For this review, take the finished solid that the model builds, in its own axes (mm). Face numbers are marked on the shaded views. Give positions to 0.01 mm unless a question says otherwise; leave off trailing zeros. Loops run counter-clockwise (first coordinate to the right, second up) from the corner with the lowest first, then second, coordinate; pieces in that order, holes last. Notation, with made-up numbers: (70.25, 44) - (85.25, 44) arc R22 ccw to (85.25, 61) - close; hole circle Ø6 at (13.25, 10.25). An arc over 180 degrees is marked (long way). Answer in a Markdown table with one row per item.
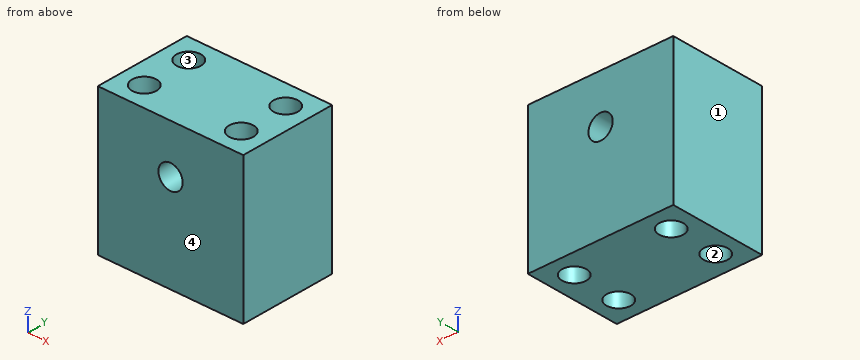
Autodesk Inventor part; units mm, degrees
ref_plane "YZ Plane" through (0, 0, 0) normal (1, 0, 0) x (0, 1, 0)
ref_plane "XZ Plane" through (0, 0, 0) normal (0, 1, 0) x (-1, 0, 0)
ref_plane "XY Plane" through (0, 0, 0) normal (0, 0, 1) x (1, 0, 0)
sketch "Sketch1" plane through (0, 0, 0) normal (0, 0, 1) x (1, 0, 0)
  line L0 (-19.05, -12.7) -> (19.05, -12.7)
  line L1 (19.05, -12.7) -> (19.05, 12.7)
  line L2 (19.05, 12.7) -> (-19.05, 12.7)
  line L3 (-19.05, 12.7) -> (-19.05, -12.7)
  line L4 (-19.05, -12.7) -> (19.05, 12.7) construction
  line L5 (19.05, -12.7) -> (-19.05, 12.7) construction
  point P0 (0, 0)
  dimension "d0" = 38.1
  dimension "d1" = 25.4
extrude "Extrusion1" add sketch "Sketch1" along normal blind 38.1
sketch "Sketch2" plane through (0, 0, 38.1) normal (0, 0, 1) x (1, 0, 0)
  line L0 (12.7, -6.35) -> (-12.7, -6.35)
  line L1 (-12.7, -6.35) -> (-12.7, 6.35)
  line L2 (-12.7, 6.35) -> (12.7, 6.35)
  line L3 (12.7, 6.35) -> (12.7, -6.35)
  line L4 (12.7, -6.35) -> (-12.7, 6.35) construction
  line L5 (-12.7, -6.35) -> (12.7, 6.35) construction
  point P0 (0, 0)
  point P1 (0, 0)
  dimension "d4" = 25.4
  dimension "d5" = 12.7
hole "Hole1" at (12.7, 6.35, 38.1) at (-12.7, 6.35, 38.1) at (-12.7, -6.35, 38.1) at (12.7, -6.35, 38.1) direction (0, 0, -1) diameter 6.35 end through all
sketch "Sketch3" plane through (-19.05, 12.7, 0) normal (0, 1, 0) x (1, 0, 0)
  line L0 (38.1, 0) -> (38.1, -38.1)
  line L1 (19.05, 0) -> (19.05, -25.4) construction
  dimension "d13" = 25.4
hole "Hole2" at (0, 12.7, 25.4) direction (0, -1, 0) diameter 6.35 end through all
properties part number "rod guide"
1. We need section D-D, the plane z = 19. Give the boundary of the cut face in (x, y) (3 decimals), and give its area (3 significant figures).
Values:
| item | result |
|---|---|
| outline | (-19.05, -12.7) - (19.05, -12.7) - (19.05, 12.7) - (-19.05, 12.7) - close; hole circle Ø6.35 at (-12.7, -6.35); hole circle Ø6.35 at (-12.7, 6.35); hole circle Ø6.35 at (12.7, -6.35); hole circle Ø6.35 at (12.7, 6.35) |
| area | 841 mm^2 |
2. We need section B-B, the plane z = 25.4. Give the boundary of the cut face in (x, y) (3 decimals), and give its area (3 significant figures).
Values:
| item | result |
|---|---|
| outline | (-19.05, -12.7) - (-3.175, -12.7) - (-3.175, 12.7) - (-19.05, 12.7) - close; (3.175, -12.7) - (19.05, -12.7) - (19.05, 12.7) - (3.175, 12.7) - close; hole circle Ø6.35 at (-12.7, -6.35); hole circle Ø6.35 at (-12.7, 6.35); hole circle Ø6.35 at (12.7, -6.35); hole circle Ø6.35 at (12.7, 6.35) |
| area | 680 mm^2 |
3. Clearance check with flat-ended pins moving along their axes: pin 1 (8 mm diameter, centred on x = 14, y = 5.5, fed in from -Z); pin 2 (4 mm diameter, centred on x = -12.7, y = -6.35, fed in from +Z). State where each tip first meets the part, or that it passes through.
Values:
| item | result |
|---|---|
| pin 1 | stops at z = 0 |
| pin 2 | passes through |
4. We need section A-A, the plane y = 6.35. Give the boundary of the cut face in (x, z) (3 decimals).
Values:
| item | result |
|---|---|
| outline | (-19.05, 0) - (-15.875, 0) - (-15.875, 38.1) - (-19.05, 38.1) - close; (-9.525, 0) - (9.525, 0) - (9.525, 38.1) - (-9.525, 38.1) - close; (15.875, 0) - (19.05, 0) - (19.05, 38.1) - (15.875, 38.1) - close; hole circle Ø6.35 at (0, 25.4) |
5. We need section C-C, the plane x = 12.7. Give the boundary of the cut face in (y, z) (3 decimals), and give its area (3 significant figures).
Values:
| item | result |
|---|---|
| outline | (-12.7, 0) - (-9.525, 0) - (-9.525, 38.1) - (-12.7, 38.1) - close; (-3.175, 0) - (3.175, 0) - (3.175, 38.1) - (-3.175, 38.1) - close; (9.525, 0) - (12.7, 0) - (12.7, 38.1) - (9.525, 38.1) - close |
| area | 484 mm^2 |
6. Wall thickness on line 1 (X direction, y = -6.35, z = 15) (3 decimals); line 2 (Y direction, x = 12.7, z = 24.5) (3 decimals); line 3 (X direction, y = -3.75, z = 2): over which ranges is each line inside the solid? List them lowest first. Write a range as [from, to].
Values:
| item | result |
|---|---|
| line 1 | x = [-19.05, -15.875], [-9.525, 9.525], [15.875, 19.05] |
| line 2 | y = [-12.7, -9.525], [-3.175, 3.175], [9.525, 12.7] |
| line 3 | x = [-19.05, -14.52], [-10.88, 10.88], [14.52, 19.05] |
7. Mouldability with a two-part tool opening along Y and no side actions: class the marked faces 1, 2, 3 and 4 as released by +Y, released by -Y, zero draft, split by the parting line, or undercut.
Values:
| item | result |
|---|---|
| face 1 | zero draft |
| face 2 | undercut |
| face 3 | undercut |
| face 4 | released by -Y |
